For this review, take the finished solid that the model builds, in its own axes (mm). Face numbers are marked on the shaded views. A direction names the side the tool comes from. Give positions to 0.01 mm unless a question says otherwise; leave off trailing zeros. Loops run counter-clockwise (first coordinate to the right, second up) from the corner with the lowest first, then second, coordinate; pieces in that order, holes last. Notation, with made-up numbers: (63.25, 51) -> (69.25, 51) arc R28 ccw to (69.25, 75) -> close; hole circle Ø2 at (-17, 62). An arc over 180 degrees is marked (long way). Answer as CSV lines item,"result". Start each with the question number.
Item 1: Clearance check with flat-ended pins moving along their axes: P1, Ø10, axis at y = -0.5, z = 11, coming from the +X side; P2, Ø1, axis at y = 22.5, z = 59, coming from the -X side; P3, Ø6.5, axis at x = 42.5, y = 17.5, coming from the +Z side; P4, Ø3, axis at x = 2.5, y = 17.5, coming from the +Z side. State where each tip first meets the part, or that it passes through.
Item 2: Add section A-A on x = -9. State the section outline as (y, z) points, plus the area to 3 significant figures.
Item 3: For L1, parallel to Y at x = 17.5, z = 86; L2, parallel to Y at x = -42.5, z = 4; L3, parallel to X at y = 14.5, z = 36.5, list the stretches that pass through material, from the lowest coordinate up. Write a range as from..to.
Item 4: Add section B-B on z = 7.5. State the section outline as (x, y) points, plus the area to 3 significant figures.
Item 5: Add section D-D on z = 42.5. State the section outline as (x, y) points, plus the area to 3 significant figures.
Item 6: Machinability: for the marked faces 1, 2 and 3, which of the approach directions +Z, -Z, +X, -X, +Y, -Y give a long, thin tool a straight path to every point of the face, cutting with its end or side? Answer none if there is none.
Item 7: Add section C-C on y = 0. State the section outline as (x, z) points, plus the area to 3 significant figures.
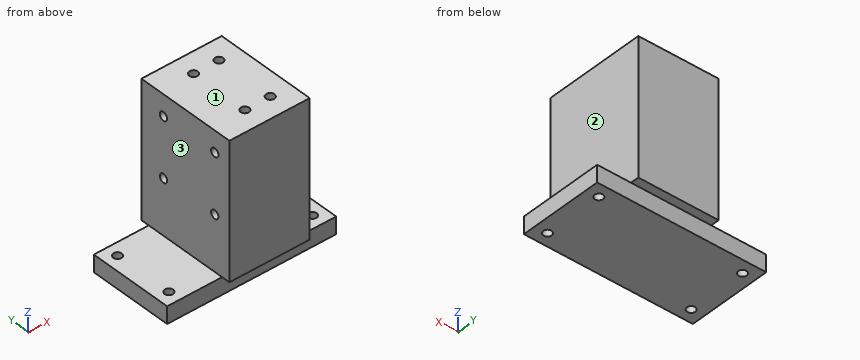
```python
from build123d import *

# Parameters (mm, degrees)
SKETCH1_W           = 100
SKETCH1_H           = 50
SKETCH1_R           = 2.5
BOSS_EXTRUDE1_DEPTH = 10
SKETCH2_W           = 47.5
SKETCH2_H           = 60
BOSS_EXTRUDE2_DEPTH = 80
SKETCH3_R           = 2.5
CUT_EXTRUDE1_DEPTH  = 10
SKETCH9_R           = 2.5
CUT_EXTRUDE18_DEPTH = 10


with BuildPart() as part:
    # Sketch1 → Boss-Extrude1 (new body)
    with BuildSketch(Plane.XY):
        Rectangle(SKETCH1_W, SKETCH1_H)
        with Locations((-42.5, 17.5)):
            Circle(SKETCH1_R, mode=Mode.SUBTRACT)
        with Locations((42.5, 17.5)):
            Circle(SKETCH1_R, mode=Mode.SUBTRACT)
        with Locations((42.5, -17.5)):
            Circle(SKETCH1_R, mode=Mode.SUBTRACT)
        with Locations((-42.5, -17.5)):
            Circle(SKETCH1_R, mode=Mode.SUBTRACT)
    extrude(amount=BOSS_EXTRUDE1_DEPTH)

    # Sketch2 → Boss-Extrude2 (add)
    with BuildSketch(Plane.XY.offset(10)):
        with Locations((6.25, 0)):
            Rectangle(SKETCH2_W, SKETCH2_H)
    extrude(amount=BOSS_EXTRUDE2_DEPTH)

    # Sketch3 → Cut-Extrude1 (cut)
    with BuildSketch(Plane.XY.offset(90)):
        with Locations((17.5, 17.5)):
            Circle(SKETCH3_R)
        with Locations((2.5, 17.5)):
            Circle(SKETCH3_R)
        with Locations((2.5, -17.5)):
            Circle(SKETCH3_R)
        with Locations((17.5, -17.5)):
            Circle(SKETCH3_R)
    extrude(amount=-CUT_EXTRUDE1_DEPTH, mode=Mode.SUBTRACT)

    # Sketch9 → Cut-Extrude18 (cut)
    with BuildSketch(Plane.ZY.offset(17.5)):
        with Locations((77.5, 15)):
            Circle(SKETCH9_R)
        with Locations((42.5, -20)):
            Circle(SKETCH9_R)
        with Locations((77.5, -20)):
            Circle(SKETCH9_R)
        with Locations((42.5, 15)):
            Circle(SKETCH9_R)
    extrude(amount=-CUT_EXTRUDE18_DEPTH, mode=Mode.SUBTRACT)


solid = part.part
```
Computed values:
1,P1,"x = 50"
1,P2,"x = -17.5"
1,P3,"z = 10"
1,P4,"z = 80"
2,outline,"(-30, 10) -> (-25, 10) -> (-25, 0) -> (25, 0) -> (25, 10) -> (30, 10) -> (30, 90) -> (-30, 90) -> close; hole circle Ø5 at (-20, 42.5); hole circle Ø5 at (-20, 77.5); hole circle Ø5 at (15, 42.5); hole circle Ø5 at (15, 77.5)"
2,area,"5,220 mm²"
3,L1,"-30..-20, -15..15, 20..30"
3,L2,"-25..-20, -15..15, 20..25"
3,L3,"-17.5..30"
4,outline,"(-50, -25) -> (50, -25) -> (50, 25) -> (-50, 25) -> close; hole circle Ø5 at (-42.5, -17.5); hole circle Ø5 at (-42.5, 17.5); hole circle Ø5 at (42.5, -17.5); hole circle Ø5 at (42.5, 17.5)"
4,area,"4,920 mm²"
5,outline,"(-17.5, -30) -> (30, -30) -> (30, 30) -> (-17.5, 30) -> (-17.5, 17.5) -> (-7.5, 17.5) -> (-7.5, 12.5) -> (-17.5, 12.5) -> (-17.5, -17.5) -> (-7.5, -17.5) -> (-7.5, -22.5) -> (-17.5, -22.5) -> close"
5,area,"2,750 mm²"
6,face 1,"+Z, +X, -X, +Y, -Y"
6,face 2,"+Z, +X, +Y, -Y"
6,face 3,"+Z, -X, +Y, -Y"
7,outline,"(-50, 0) -> (50, 0) -> (50, 10) -> (30, 10) -> (30, 90) -> (-17.5, 90) -> (-17.5, 10) -> (-50, 10) -> close"
7,area,"4,800 mm²"
